Build history of the part. All positions in model axes, mm. A direction names the side the tool comes from. Round coordinates to 2 decimals unless told otherwise and drop trailing zeros. Write each loop counter-clockwise with the first axis right and the second up, starting at its lowest first coordinate (ties: lowest second). Pieces come first, ordered by that corner, then holes. Notation, with made-up numbers: M -8,-8.75 L 1,-8.75 A20 ccw 1,17.25 Z; hole C 5,86.5 d3. An arc over 180 degrees is marked long. Write item = value, one per line. Start each with the question number.
Q1. Band-saw the part on C-C on z = 12.5. Write the cut outline in (x, y), plus the area to 3 significant figures.
Q2. Band-saw the part on D-D on x = 14. Write the cut outline in (y, z).
Q3. Pull direction X, two halves, no side cores. Call faces 4 (the flat face through (7.855, 18, 11)), 5 (the flat face through (14, 35.334, 5)), 6 (the flat face through (4, 30, 6)): released by +X, released by -X, zero draft, split by the parting line, or undercut.
Q4. Band-saw the part on B-B on y = 21. Write the cut outline in (x, z).
Q5. Probe L1, parallel to Y at x = 2.5, z = 7.25; L2, parallel to X at y = 26.5, z = 0.5; L3, parallel to Z at x = 11, y = 12. List the from-to ranges inside material, lowest first.
Q6. Tool access for faces 1 (the flat face through (22, 18, 8)), 2 (the flat face through (4, 18, 14)), 3 (the cylindrical face through (3.27, 30.47, 2.96)): list every direction of +Z, -Z, +X, -X, +Y, -Y with a clear straight run to the whole face (end or side of a thin tool).
Q7. Drop flat-ended pins along their axis: P1, Ø5, axis at x = 13.5, z = 11.5, coming from the -Y side; P2, Ø5, axis at x = 11, y = 21.5, coming from the +Z side; P3, Ø3, axis at y = 18.5, z = 10.5, coming from the +X side; P4, Ø4.5, axis at x = 3.85, y = 27.83, coming from the -Z side. Give the stop position or say it passes through.
Q8. Band-saw the part on A-A on z = 4. Write the cut outline in (x, y).
Autodesk Fusion 360 part; units mm, degrees
sketch "Sketch2" plane through (0, 0, 0) normal (0, 0, 1) x (1, 0, 0)
  line L0 (-0.1454, 35.3341) -> (35.8546, 35.3341)
  line L1 (35.8546, 35.3341) -> (35.8546, 0.3341)
  line L2 (35.8546, 0.3341) -> (-0.1454, 0.3341)
  line L3 (-0.1454, 0.3341) -> (-0.1454, 35.3341)
  line L4 (-0.1454, 17.8341) -> (35.8546, 17.8341) construction
  line L5 (23.8546, 0.3341) -> (23.8546, 35.3341) construction
  circle A0 centre (23.8546, 27.8341) radius 1.55
  circle A1 centre (23.8546, 7.8341) radius 1.55
  line L6 (3.8546, 35.3341) -> (3.8546, 0.3341) construction
  circle A2 centre (3.8546, 27.8341) radius 2
  circle A3 centre (3.8546, 7.8341) radius 2
  circle A4 centre (3.8546, 27.8341) radius 2.7
  circle A5 centre (3.8546, 7.8341) radius 2.7
  line L7 (-0.1454, 0.3341) -> (7.8546, 0.3341)
  line L8 (7.8546, 35.4069) -> (-0.1454, 35.4069)
  line L9 (-0.1454, 35.4069) -> (-0.1454, 0.3341)
  dimension "d22" = 36
  dimension "d23" = 35
  dimension "d24" = 3.1
  dimension "d25" = 3.1
  dimension "d26" = 10
  dimension "d27" = 10
  dimension "d28" = 12
  dimension "d29" = 4
  dimension "d30" = 4
  dimension "d31" = 4
  dimension "d32" = 10
  dimension "d33" = 10
  dimension "d34" = 5.4
  dimension "d35" = 5.4
  dimension "d40" = 8
extrude "Extrude5" add sketch "Sketch2" along normal blind 8 contours L0 L1 L2 L3 L7 L9 | A4 | A5
extrude "Extrude6" cut sketch "Sketch2" along normal blind 6 contours A4 | A5
sketch "Sketch3" plane through (0, 0, 8) normal (0, 0, 1) x (-1, 0, 0)
  circle A0 centre (-23.8546, -7.8341) radius 1.55
  circle A1 centre (-3.8546, -7.8341) radius 2
  circle A2 centre (-23.8546, -27.8341) radius 1.55
  circle A3 centre (-3.8546, -27.8341) radius 2
  line L0 (0.1454, -0.3341) -> (-35.8546, -0.3341)
  line L1 (-35.8546, -0.3341) -> (-35.8546, -35.3341)
  line L2 (-35.8546, -35.3341) -> (0.1454, -35.3341)
  line L3 (0.1454, -35.3341) -> (0.1454, -0.3341)
  line L4 (0.1454, -0.3341) -> (-7.8546, -0.3341)
  line L5 (-7.8546, -0.3341) -> (-7.8546, -35.3341)
  line L6 (-7.8546, -35.3341) -> (0.1454, -35.3341)
  line L7 (0.1454, -35.3341) -> (0.1454, -0.3341)
  dimension "d45" = 8
  dimension "d46" = 35
extrude "Extrude9" add sketch "Sketch3" along normal blind 6 contours L0 L2 L3 L4 L5 L6 L7
Conclusion:
q1.outline = M -0.15,0.33 L 7.85,0.33 L 7.85,35.33 L -0.15,35.33 Z; hole C 3.85,7.83 d4; hole C 3.85,27.83 d4
q1.area = 255 mm^2
q2.outline = M 0.33,0 L 35.33,0 L 35.33,8 L 0.33,8 Z
q3.face_4 = released by +X
q3.face_5 = zero draft
q3.face_6 = undercut
q4.outline = M -0.15,0 L 35.85,0 L 35.85,8 L 7.85,8 L 7.85,14 L -0.15,14 Z
q5.L1 = 0.33 to 6.36, 9.31 to 26.36, 29.31 to 35.33
q5.L2 = -0.15 to 1.51, 6.2 to 23.07, 24.64 to 35.85
q5.L3 = 0 to 8
q6.face_1 = +Z, +X, +Y, -Y
q6.face_2 = +Z, +X, -X, +Y, -Y
q6.face_3 = -Z
q7.P1 = through
q7.P2 = 8
q7.P3 = 7.85
q7.P4 = 6
q8.outline = M -0.15,0.33 L 35.85,0.33 L 35.85,35.33 L -0.15,35.33 Z; hole C 3.85,7.83 d5.4; hole C 3.85,27.83 d5.4; hole C 23.85,7.83 d3.1; hole C 23.85,27.83 d3.1
